Design review of the part built by this model. Coordinates are the model's own, in mm. Give positions to 0.01 mm unless a question says otherwise; leave off trailing zeros. Loops run counter-clockwise (first coordinate to the right, second up) from the corner with the lowest first, then second, coordinate; pieces in that order, holes last. Notation, with made-up numbers: (53.5, 79.5) -> (91.5, 79.5) arc R31 ccw to (91.5, 114.5) -> close; hole circle Ø5 at (-11, 56). An arc over 180 degrees is marked (long way). Use a Markdown table: item, result. Add a question column.
1. To check wall thickness, follow line 1 (X direction, y = 196.5, z = 0.05); line 2 (X direction, y = 196.5, z = 0.15); line 3 (Y direction, x = 20, z = 0.15). State the ranges of each line that lie inside material, in increasing order.
2. For pin 1 Ø3.5 at (x, y) = (20, 4) entering from -Z, flat-tipped, find the tip position at first contact; note if it passes through.
3. Add section B-B (y = 196.5). State the section outline as (x, z) points, and give its area (3 significant figures).
4. Add section A-A (x = 73.3). State the section outline as (y, z) points.
```python
from build123d import *

# Parameters (mm, degrees)
SKETCH_1_W          = 146.6
SKETCH_1_H          = 200
EXTRUDE_1_DEPTH     = 1.5
SKETCH_2_R          = 2
CUT_EXTRUDE_1_DEPTH = 248.979454794
CHAMFER_1_SIZE      = 1.4


with BuildPart() as part:
    # Эскиз1 → Бобышка-Вытянуть1 (new body)
    with BuildSketch(Plane.XY):
        with Locations((73.3, 100)):
            Rectangle(SKETCH_1_W, SKETCH_1_H)
    extrude(amount=EXTRUDE_1_DEPTH)

    # Эскиз2 → Вырез-Вытянуть1 (cut, through all)
    with BuildSketch(Plane.XY.offset(1.5)):
        with Locations((20, 4)):
            Circle(SKETCH_2_R)
        with Locations((20, 196.5)):
            Circle(SKETCH_2_R)
        with Locations((73.3, 196.5)):
            Circle(SKETCH_2_R)
        with Locations((73.3, 4)):
            Circle(SKETCH_2_R)
        with Locations((126.6, 196.5)):
            Circle(SKETCH_2_R)
        with Locations((126.6, 4)):
            Circle(SKETCH_2_R)
    extrude(amount=-CUT_EXTRUDE_1_DEPTH, mode=Mode.SUBTRACT)

    # Фаска1
    chamfer_1_edges = [part.edges().sort_by_distance(p)[0] for p in [
        (124.6, 4, 1.5),
        (71.3, 196.5, 1.5),
        (71.3, 4, 1.5),
        (18, 196.5, 1.5),
        (124.6, 196.5, 1.5),
        (18, 4, 1.5),
    ]]
    chamfer(chamfer_1_edges, length=CHAMFER_1_SIZE)


solid = part.part
```
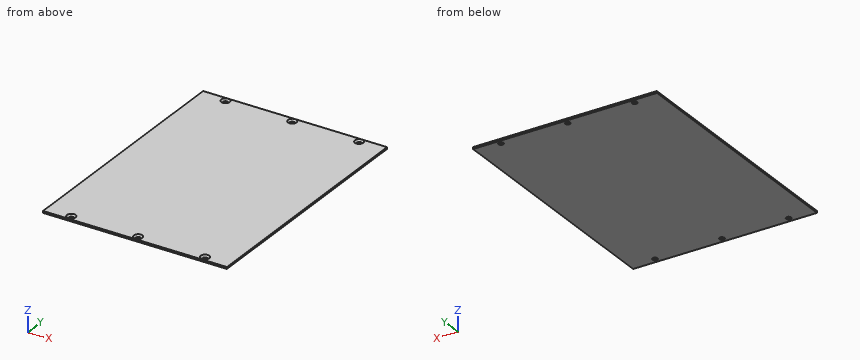
Taken from the geometry:
| question | item | result |
|---|---|---|
| 1 | line 1 | x = 0 to 18, 22 to 71.3, 75.3 to 124.6, 128.6 to 146.6 |
| 1 | line 2 | x = 0 to 17.95, 22.05 to 71.25, 75.35 to 124.55, 128.65 to 146.6 |
| 1 | line 3 | y = 0 to 1.95, 6.05 to 194.45, 198.55 to 200 |
| 2 | pin 1 | passes through |
| 3 | outline | (0, 0) -> (18, 0) -> (18, 0.1) -> (16.6, 1.5) -> (0, 1.5) -> close; (22, 0) -> (71.3, 0) -> (71.3, 0.1) -> (69.9, 1.5) -> (23.4, 1.5) -> (22, 0.1) -> close; (75.3, 0) -> (124.6, 0) -> (124.6, 0.1) -> (123.2, 1.5) -> (76.7, 1.5) -> (75.3, 0.1) -> close; (128.6, 0) -> (146.6, 0) -> (146.6, 1.5) -> (130, 1.5) -> (128.6, 0.1) -> close |
| 3 | area | 196 mm^2 |
| 4 | outline | (0, 0) -> (2, 0) -> (2, 0.1) -> (0.6, 1.5) -> (0, 1.5) -> close; (6, 0) -> (194.5, 0) -> (194.5, 0.1) -> (193.1, 1.5) -> (7.4, 1.5) -> (6, 0.1) -> close; (198.5, 0) -> (200, 0) -> (200, 1.5) -> (199.9, 1.5) -> (198.5, 0.1) -> close |
